from build123d import *

# Parameters (mm, degrees)
SKETCH1_W           = 17.78
SKETCH1_H           = 38.1
SKETCH1_R           = 3.683
BOSS_EXTRUDE1_DEPTH = 12.7
SKETCH2_W           = 12.7
SKETCH2_H           = 2.54
BOSS_EXTRUDE2_DEPTH = 15.24
SKETCH3_W           = 12.7
SKETCH3_H           = 2.54
BOSS_EXTRUDE3_DEPTH = 15.24
SKETCH4_R           = 3.429
CUT_EXTRUDE1_DEPTH  = 52.992503306


with BuildPart() as part:
    # Sketch1 → Boss-Extrude1 (new body)
    with BuildSketch(Plane.XY):
        with Locations((8.89, 19.05)):
            Rectangle(SKETCH1_W, SKETCH1_H)
        with Locations((8.89, 30.988)):
            Circle(SKETCH1_R, mode=Mode.SUBTRACT)
        with Locations((8.89, 21.209)):
            Circle(SKETCH1_R, mode=Mode.SUBTRACT)
        with Locations((8.89, 11.43)):
            Circle(SKETCH1_R, mode=Mode.SUBTRACT)
    extrude(amount=BOSS_EXTRUDE1_DEPTH)

    # Sketch2 → Boss-Extrude2 (add)
    with BuildSketch(Plane(origin=(17.78, 0, 0), x_dir=(0, 0, -1), z_dir=(1, 0, 0))):
        with Locations((-6.35, 1.27)):
            Rectangle(SKETCH2_W, SKETCH2_H)
    extrude(amount=BOSS_EXTRUDE2_DEPTH)

    # Sketch3 → Boss-Extrude3 (add)
    with BuildSketch(Plane.ZY):
        with Locations((6.35, 1.27)):
            Rectangle(SKETCH3_W, SKETCH3_H)
    extrude(amount=BOSS_EXTRUDE3_DEPTH)

    # Sketch4 → Cut-Extrude1 (cut, through all)
    with BuildSketch(Plane.XZ):
        with Locations(Location((-6.985, 6.35, 0), (0, 0, 270))):
            Circle(SKETCH4_R)
        with Locations(Location((24.765, 6.35, 0), (0, 0, 270))):
            Circle(SKETCH4_R)
    extrude(amount=-CUT_EXTRUDE1_DEPTH, mode=Mode.SUBTRACT)


solid = part.part
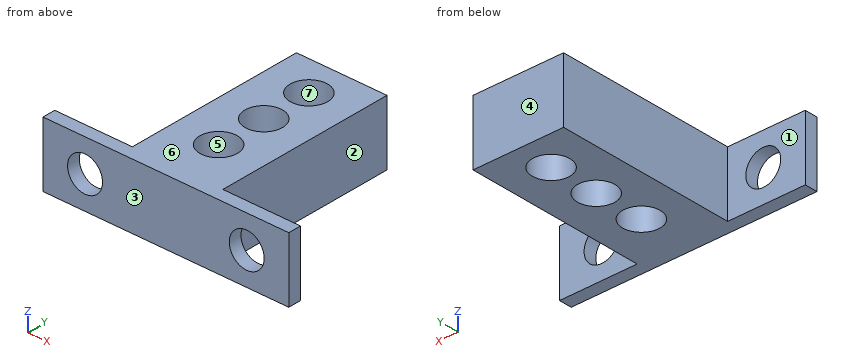
The model under review builds one solid part; all positions refer to its coordinate system, in mm. Face numbers are marked on the shaded views. A direction names the side the tool comes from. Round coordinates to 2 decimals unless told otherwise and drop trailing zeros. Order: outer loops, then holes, each group sorted by start corner. A loop starts at its lowest first (then second) coordinate and runs counter-clockwise, first axis right, second up. Notation, with made-up numbers: (50.5, -26) -> (107.5, -26) arc R9 ccw to (107.5, -16) -> close; hole circle Ø10 at (58.5, 52). An arc over 180 degrees is marked (long way). Write item = value, one per line. Start each with the question number.
Item 1: For the marked faces 1, 2 and 3, list the 3-axis set-ups (+Z, -Z, +X, -X, +Y, -Y) from which the entire face can be reached by the end or side of a thin tool; tool diameter is ignored.
Item 2: Consider section C-C on y = 32. Write out the cut boundary in (x, z).
Item 3: Clearance check with flat-ended pins moving along their axes: pin 1 Ø1 at (y, z) = (27, 2.5) entering from +X; pin 2 Ø6.5 at (y, z) = (25.5, 9) entering from -X; pin 3 Ø1.5 at (x, z) = (24, 9) entering from +Y. State where each tip first meets the part, or that it passes through.
Item 4: Consider section B-B on x = 8.89. Write out the cut boundary in (y, z) (3 decimals), plus the area to 3 significant figures.
Item 5: Mouldability with a two-part tool opening along Y and no side actions: class the marked faces 4, 5, 6 and 7 as released by +Y, released by -Y, zero draft, split by the parting line, or undercut.
Item 6: Consider section A-A on z = 6.35. Write out the cut boundary in (x, y), plus the area to 3 significant figures.
Item 7: For line 1 along X through (y, z) = (0.6, 6.35); line 2 along Y through (x, z) = (8.89, 6.75) (3 decimals); line 3 along X through (y, z) = (31, 1), list the stretches that pass through material, from the lowest coordinate up.
Item 8: Consider section D-D on y = 11.43. Write out the cut boundary in (x, z), plus the area to 3 significant figures.
Conclusion:
q1.face_1 = +Z, -Z, -X, +Y
q1.face_2 = +Z, -Z, +X, +Y
q1.face_3 = +Z, -Z, +X, -X, -Y
q2.outline = (0, 0) -> (5.35, 0) -> (5.35, 12.7) -> (0, 12.7) -> close; (12.43, 0) -> (17.78, 0) -> (17.78, 12.7) -> (12.43, 12.7) -> close
q3.pin_1 = 17.78
q3.pin_2 = 0
q3.pin_3 = 2.54
q4.outline = (0, 0) -> (7.747, 0) -> (7.747, 12.7) -> (0, 12.7) -> close; (15.113, 0) -> (17.526, 0) -> (17.526, 12.7) -> (15.113, 12.7) -> close; (24.892, 0) -> (27.305, 0) -> (27.305, 12.7) -> (24.892, 12.7) -> close; (34.671, 0) -> (38.1, 0) -> (38.1, 12.7) -> (34.671, 12.7) -> close
q4.area = 203 mm2
q5.face_4 = released by +Y
q5.face_5 = undercut
q5.face_6 = zero draft
q5.face_7 = undercut
q6.outline = (-15.24, 0) -> (-10.41, 0) -> (-10.41, 2.54) -> (-15.24, 2.54) -> close; (-3.56, 0) -> (21.34, 0) -> (21.34, 2.54) -> (17.78, 2.54) -> (17.78, 38.1) -> (0, 38.1) -> (0, 2.54) -> (-3.56, 2.54) -> close; (28.19, 0) -> (33.02, 0) -> (33.02, 2.54) -> (28.19, 2.54) -> close; hole circle Ø7.37 at (8.89, 11.43); hole circle Ø7.37 at (8.89, 21.21); hole circle Ø7.37 at (8.89, 30.99)
q6.area = 592 mm2
q7.line_1 = -15.24 to -10.41, -3.56 to 21.34, 28.19 to 33.02
q7.line_2 = 0 to 7.747, 15.113 to 17.526, 24.892 to 27.305, 34.671 to 38.1
q7.line_3 = 0 to 5.21, 12.57 to 17.78
q8.outline = (0, 0) -> (5.21, 0) -> (5.21, 12.7) -> (0, 12.7) -> close; (12.57, 0) -> (17.78, 0) -> (17.78, 12.7) -> (12.57, 12.7) -> close
q8.area = 132 mm2
